Can you work these out from the model? Positions are in its coordinate system, mm. Round coordinates to 2 decimals unless told otherwise and drop trailing zeros. Order: outer loops, then holes, each group sorted by start corner. A loop starts at its lowest first (then second) coordinate and runs counter-clockwise, first axis right, second up. Notation, with made-up numbers: (-37, 79) -> (15, 79) arc R26 ccw to (15, 97) -> close; hole circle Ø8 at (20.25, 76.25). An arc over 180 degrees is marked (long way). Use a Markdown table: item, result. Add a question column.
Q1. I'm going to push flat-ended pins straight in: pin 1 Ø5 at (y, z) = (142, 22.5) entering from -X; pin 2 Ø1.5 at (y, z) = (157, 35.5) entering from -X; pin 3 Ø12 at (x, z) = (-110, 18) entering from +Y. Where does each tip first touch, or does it pass through?
Q2. If we section it at B-B on y = 170: List the corners of the cut face in (x, z) for me, plus the area to 3 significant figures.
Q3. If we section it at A-A on z = 36: List the corners of the cut face in (x, y) for me.
Q4. I need wall thicknesses on line 1 along X through (y, z) = (259.5, 17.5); line 2 along X through (y, z) = (82, 18); line 3 along Y through (x, z) = (-34, 30). Which ranges of each line are inside material? Lowest first, please. Write a range as [from, to].
Q5. We'd pull the mould along Z, two halves only. Please class faces 1 (the face through (-223.3, 170.87, 24.78)), 2 (the face through (-224, 176, 9)), 3 (the face through (-161.53, 131.23, 29.06)), 4 (the face through (-224, 176, 41)): +Z half, -Z half, draft (parallel to the pull), parting line (faces both ways), or undercut.
```python
from build123d import *

# Parameters (mm, degrees)
PAD006_DEPTH           = 32
SKETCH014_R            = 6
POCKET004_DEPTH        = 273.736822
LINEARPATTERN002_COUNT = 4
LINEARPATTERN002_PITCH = 173.333333


with BuildPart() as part:
    # Sketch013 → Pad006 (new body)
    with BuildSketch(Plane.XY):
        Polygon((-456.521681, 341.5), (10.26148, 14.654912), (6.820021, 9.74), (-459.963139, 336.585088), align=None)
    extrude(amount=PAD006_DEPTH)

    # Sketch014 (on Face3 of Pad006) → Pocket004 (cut, through all)
    with BuildSketch(Plane(origin=(6.820021, 9.74, 0), x_dir=(0.819152, -0.573576, 0), z_dir=(-0.573576, -0.819152, 0))):
        with Locations((-549.837021, 16)):
            Circle(SKETCH014_R)
    pocket004 = extrude(amount=-POCKET004_DEPTH, mode=Mode.SUBTRACT)

    # LinearPattern002: Pocket004 ×4
    with Locations(*[Vector(0.819152, -0.573576, 0) * (i * LINEARPATTERN002_PITCH) for i in range(1, LINEARPATTERN002_COUNT)]):
        add(pocket004, mode=Mode.SUBTRACT)


with BuildPart() as part_1:
    # Body005 placement: moved
    add(part.part.moved(Location((0, 0, 9))))


solid = part_1.part
```
Answer below:
| question | item | result |
|---|---|---|
| 1 | pin 1 | x = -185.64 |
| 1 | pin 2 | x = -204.56 |
| 1 | pin 3 | y = 103.06 |
| 2 | outline | (-222.05, 9) -> (-211.59, 9) -> (-211.59, 41) -> (-222.05, 41) -> close |
| 2 | area | 335 mm² |
| 3 | outline | (-459.96, 336.59) -> (6.82, 9.74) -> (10.26, 14.65) -> (-456.52, 341.5) -> close |
| 4 | line 1 | [-349.87, -339.41] |
| 4 | line 2 | [-96.38, -85.92] |
| 4 | line 3 | [38.32, 45.65] |
| 5 | face 1 | draft |
| 5 | face 2 | -Z half |
| 5 | face 3 | undercut |
| 5 | face 4 | +Z half |
